Read the model definition and answer for the solid it produces. Units are mm, in the model's axes. A direction names the side the tool comes from. Coordinates: 2 decimals unless noted, no trailing zeros. Loops run counter-clockwise (first coordinate to the right, second up) from the corner with the lowest first, then second, coordinate; pieces in that order, holes last.
Q1. Section B-B (y = 26.5) is taken. Give the vertices of the cut face in (x, z), then the cut area to 3 significant figures.
Q2. Section A-A (y = 36.15) is taken. Give the vertices of the cut face in (x, z), then the cut area to 3 significant figures.
Q3. Section C-C (x = -22.5) is taken. Give the vertices of the cut face in (y, z).
Q4. Straight lines are drawn through the part: line 1 (X direction, y = 6.75, z = 0); line 2 (Y direction, x = 15, z = 0); line 3 (X direction, y = 34, z = -7). For each, find the intervals that lie inside material, in ascending order.
Q5. Flat-ended cylindrical pins translate along their axes: P1, Ø6, axis at y = 30.5, z = 5, coming from the -X side; P2, Ø5, axis at x = 22.5, z = 0, coming from the +Y side; P3, Ø1, axis at y = 13.5, z = -2.5, coming from the +X side. Find the tip coordinate at first contact, or state that the pin passes through.
Q6. The mould has two halves that part along X. Classify faces 4 (the face through (-25, 10, 0)), 5 (the face through (-27.5, 5, 0)), 6 (the face through (10.1, 43.58, -0.14)): pulls with the +X half, pulls with the -X half, needs draft (parallel to the pull), parting line crosses it, or undercut.
Q7. Which of the six approach directions +Z, -Z, +X, -X, +Y, -Y give full straight-line access (tool end or side, diameter ignored) to faces 1 (the face through (25, 10, 0)), 2 (the face through (-14, 44.15, 0)), 3 (the face through (8.93, 14.75, -0.14))?
Q8. Section D-D (z = 5.25) is taken. Give the vertices of the cut face in (x, y), then the cut area to 3 significant figures.
from build123d import *

# Parameters (mm, degrees)
SKETCH1_W               = 35
SKETCH1_H               = 20
BOSS_EXTRUDE1_DEPTH     = 44.15
SKETCH2_W               = 19
SKETCH2_H               = 20
CUT_EXTRUDE1_DEPTH      = 30
CUT_EXTRUDE2_DEPTH      = 58.220822259
CUT_EXTRUDE2_DEPTH_BACK = 58.220822259
SKETCH3_R               = 2.5
FILLET1_R               = 2
SKETCH4_W               = 10
SKETCH4_H               = 20
SKETCH4_R               = 2
BOSS_EXTRUDE2_DEPTH     = 10
FILLET2_R               = 2


with BuildPart() as part:
    # Sketch1 → Boss-Extrude1 (new body)
    with BuildSketch(Plane(origin=(0, 0, 0), x_dir=(1, 0, 0), z_dir=(0, 1, 0))):
        Rectangle(SKETCH1_W, SKETCH1_H)
    extrude(amount=BOSS_EXTRUDE1_DEPTH)

    # Sketch2 → Cut-Extrude1 (cut)
    with BuildSketch(Plane(origin=(0, 44.15, 0), x_dir=(1, 0, 0), z_dir=(0, 1, 0))):
        Rectangle(SKETCH2_W, SKETCH2_H)
    extrude(amount=-CUT_EXTRUDE1_DEPTH, mode=Mode.SUBTRACT)

    # Sketch3 → Cut-Extrude2 (cut, two sides: drawn at the far end of the back side and taken through both)
    with BuildSketch(Plane(origin=(17.5, 0, 0), x_dir=(0, 0, -1), z_dir=(1, 0, 0)).offset(-CUT_EXTRUDE2_DEPTH_BACK)):
        with Locations((0, 36.15)):
            Circle(SKETCH3_R)
    extrude(amount=CUT_EXTRUDE2_DEPTH + CUT_EXTRUDE2_DEPTH_BACK, mode=Mode.SUBTRACT)

    # Fillet1
    fillet1_edges = [part.edges().sort_by_distance(p)[0] for p in [
        (9.5, 14.15, 0),
        (-9.5, 14.15, 0),
        (9.5, 44.15, 0),
        (-9.5, 44.15, 0),
    ]]
    fillet(fillet1_edges, radius=FILLET1_R)

    # Sketch4 → Boss-Extrude2 (add)
    # profile 1 of 2: a face of its own
    with BuildSketch(Plane.XZ):
        with Locations((22.5, 0)):
            Rectangle(SKETCH4_W, SKETCH4_H)
        with Locations(Location((22.5, 0, 0), (0, 0, 270))):
            Circle(SKETCH4_R, mode=Mode.SUBTRACT)
    # profile 2 of 2: a face of its own
    with BuildSketch(Plane.XZ):
        with Locations((-22.5, 0)):
            Rectangle(SKETCH4_W, SKETCH4_H)
        with Locations(Location((-22.5, 0, 0), (0, 0, 90))):
            Circle(SKETCH4_R, mode=Mode.SUBTRACT)
    extrude(amount=-BOSS_EXTRUDE2_DEPTH)

    # Fillet2
    fillet2_edges = [part.edges().sort_by_distance(p)[0] for p in [
        (-17.5, 44.15, 0),
        (17.5, 44.15, 0),
        (17.5, 10, 0),
        (-17.5, 10, 0),
    ]]
    fillet(fillet2_edges, radius=FILLET2_R)


solid = part.part
Numbers:
1. outline: (-17.5, -10) - (-9.5, -10) - (-9.5, 10) - (-17.5, 10) - close; (9.5, -10) - (17.5, -10) - (17.5, 10) - (9.5, 10) - close
1. area: 320 mm2
2. outline: (-17.5, -10) - (-9.5, -10) - (-9.5, -2.5) - (-17.5, -2.5) - close; (-17.5, 2.5) - (-9.5, 2.5) - (-9.5, 10) - (-17.5, 10) - close; (9.5, -10) - (17.5, -10) - (17.5, -2.5) - (9.5, -2.5) - close; (9.5, 2.5) - (17.5, 2.5) - (17.5, 10) - (9.5, 10) - close
2. area: 240 mm2
3. outline: (0, -10) - (10, -10) - (10, -2) - (0, -2) - close; (0, 2) - (10, 2) - (10, 10) - (0, 10) - close
4. line 1: x = -27.5 to -24.5, -20.5 to 20.5, 24.5 to 27.5
4. line 2: y = 0 to 33.65, 38.65 to 44.15
4. line 3: x = -17.5 to -9.5, 9.5 to 17.5
5. P1: stops at x = -17.5
5. P2: stops at y = 10
5. P3: stops at x = 17.5
6. face 4: needs draft
6. face 5: pulls with the -X half
6. face 6: undercut
7. face 1: +Z, -Z, +X, +Y
7. face 2: +Z, -Z, +X, -X, +Y
7. face 3: +Z, -Z, +Y
8. outline: (-27.5, 0) - (27.5, 0) - (27.5, 10) - (19.5, 10) arc R2 cw to (17.5, 12) - (17.5, 42.15) arc R2 ccw to (15.5, 44.15) - (11.5, 44.15) arc R2 ccw to (9.5, 42.15) - (9.5, 16.15) arc R2 cw to (7.5, 14.15) - (-7.5, 14.15) arc R2 cw to (-9.5, 16.15) - (-9.5, 42.15) arc R2 ccw to (-11.5, 44.15) - (-15.5, 44.15) arc R2 ccw to (-17.5, 42.15) - (-17.5, 12) arc R2 cw to (-19.5, 10) - (-27.5, 10) - close
8. area: 1,180 mm2
